Geometry: final body of the model. Coordinates: model frame, mm. A direction names the side the tool comes from. Coordinates: 2 decimals unless noted, no trailing zeros. Loops run counter-clockwise (first coordinate to the right, second up) from the corner with the lowest first, then second, coordinate; pieces in that order, holes last. Notation, with made-up numbers: M -9,10.5 L -3,10.5 A17 ccw -3,20.5 Z; hole C -20,-7.75 d10. An arc over 180 degrees is marked long. Write each question's results on one line, items separated by ' | '. Start each with the question number.
from build123d import *

# Parameters (mm, degrees)
SKETCH_1_W          = 101
SKETCH_1_H          = 55.5
SKETCH_1_W_2        = 91
SKETCH_1_H_2        = 45.5
EXTRUDE_1_DEPTH     = 50
SKETCH_2_W          = 101
SKETCH_2_H          = 55.5
EXTRUDE_2_DEPTH     = 5
SKETCH_4_W          = 101
SKETCH_4_H          = 3
EXTRUDE_3_DEPTH     = 2
SKETCH_7_W          = 91
SKETCH_7_H          = 5.5
CUT_EXTRUDE_1_DEPTH = 3
SKETCH_9_W          = 40
SKETCH_9_H          = 9
CUT_EXTRUDE_2_DEPTH = 3
CUT_EXTRUDE_3_DEPTH = 10
CUT_EXTRUDE_4_DEPTH = 106
EXTRUDE_4_DEPTH     = 100
SKETCH_13_R         = 4
CUT_EXTRUDE_5_DEPTH = 137
SKETCH_14_R         = 3
SKETCH_14_R_2       = 1.5
EXTRUDE_5_DEPTH     = 3
CUT_EXTRUDE_START   = -2
SKETCH_14_3_R       = 1.5
CUT_EXTRUDE_6_DEPTH = 2
EXTRUDE_6_DEPTH     = 3
EXTRUDE_7_DEPTH     = 10
EXTRUDE_9_REACH     = 100.647
EXTRUDE_8_REACH     = 88.283
SKETCH_18_W         = 3
SKETCH_18_H         = 3
SKETCH_19_W         = 5
SKETCH_19_H         = 1.94594374
CUT_EXTRUDE_7_DEPTH = 13
EXTRUDE_10_REACH    = 119.48
EXTRUDE_11_DEPTH    = 86


with BuildPart() as part:
    # 草图1 → 凸台-拉伸1 (new body)
    with BuildSketch(Plane.XY):
        Rectangle(SKETCH_1_W, SKETCH_1_H)
        Rectangle(SKETCH_1_W_2, SKETCH_1_H_2, mode=Mode.SUBTRACT)
    extrude(amount=EXTRUDE_1_DEPTH)

    # 草图2 → 凸台-拉伸2 (add)
    with BuildSketch(Plane.XY):
        Rectangle(SKETCH_2_W, SKETCH_2_H)
    extrude(amount=-EXTRUDE_2_DEPTH)

    # 草图4 → 凸台-拉伸3 (add)
    with BuildSketch(Plane.XZ.offset(-22.75)):
        with Locations((0, 38.5)):
            Rectangle(SKETCH_4_W, SKETCH_4_H)
    extrude(amount=EXTRUDE_3_DEPTH)

    # 草图7 → 切除-拉伸1 (cut)
    with BuildSketch(Plane(origin=(0, -22.75, 0), x_dir=(1, 0, 0), z_dir=(0, 1, 0))):
        with Locations((0, -45.25)):
            Rectangle(SKETCH_7_W, SKETCH_7_H)
    extrude(amount=-CUT_EXTRUDE_1_DEPTH, mode=Mode.SUBTRACT)

    # 草图9 → 切除-拉伸2 (cut)
    with BuildSketch(Plane.XY):
        with Locations((0.5, 18.25)):
            Rectangle(SKETCH_9_W, SKETCH_9_H)
    extrude(amount=-CUT_EXTRUDE_2_DEPTH, mode=Mode.SUBTRACT)

    # 草图10 → 切除-拉伸3 (cut)
    with BuildSketch(Plane(origin=(0, 0, -5), x_dir=(-1, 0, 0), z_dir=(0, 0, -1))):
        with BuildLine():
            Line((-4.5, 18.75), (4.5, 18.75))
            ThreePointArc((4.5, 18.75), (7, 16.25), (4.5, 13.75))
            Line((4.5, 13.75), (-4.5, 13.75))
            ThreePointArc((-4.5, 13.75), (-7, 16.25), (-4.5, 18.75))
        make_face()
    extrude(amount=-CUT_EXTRUDE_3_DEPTH, mode=Mode.SUBTRACT)

    # 草图11 → 切除-拉伸4 (cut)
    with BuildSketch(Plane(origin=(50.5, 0, 0), x_dir=(0, 0, -1), z_dir=(1, 0, 0))):
        Polygon((-50, -27.75), (5, -20.020254091), (5, -27.75), align=None)
    extrude(amount=-CUT_EXTRUDE_4_DEPTH, mode=Mode.SUBTRACT)

    # 草图12 → 凸台-拉伸4 (add)
    with BuildSketch(Plane(origin=(50.5, 0, 0), x_dir=(0, 0, -1), z_dir=(1, 0, 0))):
        Polygon((5, -20.020254091), (5, -18.020254091), (-50, -25.75), (-50, -27.75), align=None)
    extrude(amount=-EXTRUDE_4_DEPTH)

    # 草图13 → 切除-拉伸5 (cut)
    with BuildSketch(Plane(origin=(0, 0, 0), x_dir=(1, 0, 0), z_dir=(0, 1, 0))):
        with Locations(Location((-12.5, -9.5, 0), (0, 0, 90))):
            Circle(SKETCH_13_R)
        with Locations(Location((12.55, -9.5, 0), (0, 0, 90))):
            Circle(SKETCH_13_R)
    extrude(amount=-CUT_EXTRUDE_5_DEPTH, mode=Mode.SUBTRACT)

    # 草图14 → 凸台-拉伸5 (add)
    # profile 1 of 2: a face of its own
    with BuildSketch(Plane.XZ.offset(-22.75)):
        with Locations(Location((-12.5, 9.5, 0), (0, 0, 270))):
            Circle(SKETCH_14_R)
        with Locations(Location((-12.5, 9.5, 0), (0, 0, 270))):
            Circle(SKETCH_14_R_2, mode=Mode.SUBTRACT)
    # profile 2 of 2: a face of its own
    with BuildSketch(Plane.XZ.offset(-22.75)):
        with Locations(Location((12.55, 9.5, 0), (0, 0, 270))):
            Circle(SKETCH_14_R)
        with Locations(Location((12.55, 9.5, 0), (0, 0, 270))):
            Circle(SKETCH_14_R_2, mode=Mode.SUBTRACT)
    extrude(amount=EXTRUDE_5_DEPTH)

    # 草图14<3> → 切除-拉伸6 (cut)
    with BuildSketch(Plane.XZ.offset(-22.75).offset(CUT_EXTRUDE_START)):
        with Locations(Location((-12.5, 9.5, 0), (0, 0, 270))):
            Circle(SKETCH_14_3_R)
        with Locations(Location((12.55, 9.5, 0), (0, 0, 270))):
            Circle(SKETCH_14_3_R)
    extrude(amount=CUT_EXTRUDE_6_DEPTH, mode=Mode.SUBTRACT)

    # 草图15 → 凸台-拉伸6 (add)
    with BuildSketch(Plane.XY.offset(40)):
        Polygon((-45.5, 20.75), (-43.5, 20.75), (-43.5, -20.75), (43.5, -20.75), (43.5, 20.75), (45.5, 20.75), (45.5, -22.75), (43.3124719, -22.75), (-43.5, -22.75), (-45.5, -22.75), align=None)
    extrude(amount=-EXTRUDE_6_DEPTH)

    # 草图17 → 凸台-拉伸7 (add)
    with BuildSketch(Plane(origin=(50.5, 0, 0), x_dir=(0, 0, -1), z_dir=(1, 0, 0))):
        Polygon((-50, -27.75), (-50, -45.66717529), (5, -20.020254091), align=None)
    extrude_7 = extrude(amount=-EXTRUDE_7_DEPTH)

    # 镜向1: 凸台-拉伸7 across plane
    add(extrude_7.mirror(Plane(origin=(0, 0, 0), x_dir=(0, 0, 1), z_dir=(1, 0, 0))))

    # 草图21 → 凸台-拉伸9 (add, up to next)
    with BuildSketch(Plane.XZ.offset(-22.75), mode=Mode.PRIVATE) as extrude_9_sk1:
        Polygon((-45.5, 34), (-45.5, 37), (-43.5, 37), align=None)
    extrude_9_tool1 = extrude(extrude_9_sk1.sketch, amount=EXTRUDE_9_REACH, mode=Mode.PRIVATE) - part.part
    extrude_9 = extrude_9_tool1.solids().sort_by_distance((-44.833333, 22.75, 36))[0]
    add(extrude_9)

    # 镜向2: 凸台-拉伸9 across plane
    add(extrude_9.mirror(Plane(origin=(0, 0, 0), x_dir=(0, 0, 1), z_dir=(1, 0, 0))))

    # 草图18 → 凸台-拉伸8 (add, up to next)
    with BuildSketch(Plane.XY.offset(-3), mode=Mode.PRIVATE) as extrude_8_sk1:
        with Locations((-12.5, 21.25)):
            Rectangle(SKETCH_18_W, SKETCH_18_H)
    extrude_8_tool1 = extrude(extrude_8_sk1.sketch, amount=EXTRUDE_8_REACH, mode=Mode.PRIVATE) - part.part
    # 草图18 → 凸台-拉伸8 (add, up to next)
    with BuildSketch(Plane.XY.offset(-3), mode=Mode.PRIVATE) as extrude_8_sk2:
        with Locations((12.55, 21.25)):
            Rectangle(SKETCH_18_W, SKETCH_18_H)
    extrude_8_tool2 = extrude(extrude_8_sk2.sketch, amount=EXTRUDE_8_REACH, mode=Mode.PRIVATE) - part.part
    add(extrude_8_tool1.solids().sort_by_distance((-12.5, 21.25, -3))[0])
    add(extrude_8_tool2.solids().sort_by_distance((12.55, 21.25, -3))[0])

    # 草图19 → 切除-拉伸7 (cut)
    with BuildSketch(Plane.XY.offset(42.5)):
        with Locations((43, -23.72297187)):
            Rectangle(SKETCH_19_W, SKETCH_19_H)
    extrude(amount=-CUT_EXTRUDE_7_DEPTH, mode=Mode.SUBTRACT)

    # 凸台-拉伸10: up to this plane
    extrude_10_end = Plane(origin=(-43.5, -45.66917529, 37), z_dir=(-0.8320502943378437, 0, 0.5547001962252291))
    # 草图23 → 凸台-拉伸10 (add, up to the surface)
    with BuildSketch(Plane.ZY.offset(-45.5), mode=Mode.PRIVATE) as extrude_10_sk1:
        Polygon((34, 22.75), (37, 22.75), (37, 20.75), align=None)
    extrude_10_tool1 = split(extrude(extrude_10_sk1.sketch, amount=EXTRUDE_10_REACH, mode=Mode.PRIVATE), bisect_by=extrude_10_end, keep=Keep.BOTH, mode=Mode.PRIVATE)
    add(extrude_10_tool1.solids().sort_by_distance((45.5, 22.083333, 36))[0])

    # 草图24 → 凸台-拉伸11 (add)
    with BuildSketch(Plane(origin=(-45.5, 0, 0), x_dir=(0, 0, -1), z_dir=(1, 0, 0))):
        Polygon((-34, -22.75), (-37, -22.75), (-37, -20.75), align=None)
    extrude(amount=EXTRUDE_11_DEPTH)


solid = part.part
Item 1: Set-up query: faces 1 (the flat face through (-1, -20.75, 39)), 2 (the flat face through (40.5, -24, 36)), 3 (the cylindrical face through (-7, 16.3, -4)), 4 (the cylindrical face through (-12.43, 22.28, 11)), 5 (the flat face through (40.5, -33, 29)). Return all of +Z, -Z, +X, -X, +Y, -Y with unobstructed straight access to the full face (end or side cutting, diameter ignored); none if empty.
Item 2: Section C-C, the plane z = 44. Return loops of the section in (x, y).
Item 3: Contact query for flat-ended pins moving along their axis: P1, Ø4, axis at x = -4.5, z = 27.5, coming from the -Y side; P2, Ø13, axis at x = -12.5, z = 9.5, coming from the -Y side; P3, Ø1.5, axis at x = 12.5, z = 38, coming from the -Y side. Output: stop coordinate, or through.
Item 4: Pull-direction query (Y, two-part tool) for faces 6 (the cylindrical face through (16.455, -21.062, 10.367)), 7 (the flat face through (-1, -24, 48)); classes: released by +Y, released by -Y, zero draft, split by the parting line, or undercut.
Item 5: Section D-D, the plane y = -31.5. Return loops of the section in (x, z), plus the area to 3 significant figures.
Item 6: Section B-B, the plane y = -3.5. Return loops of the section in (x, z).
Item 7: Ray query, L1, parallel to X at y = -21.7, z = 9.5; L2, parallel to X at y = 23.1, z = 9.5; L3, parallel to X at y = 12, z = 25.5. Return the intervals inside material, ascending. Write a range as [from, to].
Solutions:
1) face 1: +Z | face 2: none | face 3: +Z, -Z | face 4: -Y | face 5: -Z, -Y
2) outline: M -50.5,-42.87 L -40.5,-42.87 L -40.5,-26.91 L 40.5,-26.91 L 40.5,-42.87 L 50.5,-42.87 L 50.5,27.75 L -50.5,27.75 Z; hole M -45.5,-24.91 L 45.5,-24.91 L 45.5,22.75 L -45.5,22.75 Z
3) P1: stops at y = -24.87 | P2: stops at y = -22.97 | P3: stops at y = -26.17
4) face 6: zero draft | face 7: undercut
5) outline: M -50.5,19.62 L -40.5,19.62 L -40.5,50 L -50.5,50 Z; M 40.5,19.62 L 50.5,19.62 L 50.5,50 L 40.5,50 Z | area: 608 mm²
6) outline: M -50.5,-5 L 50.5,-5 L 50.5,50 L 45.5,50 L 45.5,40 L 43.5,40 L 43.5,37 L 45.5,34 L 45.5,0 L -45.5,0 L -45.5,34 L -43.5,37 L -43.5,40 L -45.5,40 L -45.5,50 L -50.5,50 Z
7) L1: x = [-50.5, -16.5], [-8.5, 8.55], [16.55, 50.5] | L2: x = [-50.5, -14], [-11, 11.05], [14.05, 50.5] | L3: x = [-50.5, -45.5], [45.5, 50.5]
